```python
from build123d import *

# Parameters (mm, degrees)
SKETCH1_R                = 50
BOSS_EXTRUDE1_DEPTH      = 10
SKETCH2_R                = 20
BOSS_EXTRUDE2_DEPTH      = 280
BOSS_EXTRUDE3_START      = -10
BOSS_EXTRUDE3_DEPTH      = 10
BOSS_EXTRUDE4_DEPTH      = 10
BOSS_EXTRUDE4_DEPTH_BACK = 10
SKETCH5_R                = 20


with BuildPart() as part:
    # Sketch1 → Boss-Extrude1 (new body)
    with BuildSketch(Plane(origin=(0, 0, 0), x_dir=(1, 0, 0), z_dir=(0, 1, 0))):
        with Locations(Location((0, 0, 0), (0, 0, 270))):
            Circle(SKETCH1_R)
    extrude(amount=BOSS_EXTRUDE1_DEPTH)

    # Sketch2 → Boss-Extrude2 (add)
    with BuildSketch(Plane(origin=(0, 10, 0), x_dir=(1, 0, 0), z_dir=(0, 1, 0))):
        with Locations(Location((0, 0, 0), (0, 0, 270))):
            Circle(SKETCH2_R)
    extrude(amount=BOSS_EXTRUDE2_DEPTH)

    # Sketch4 → Boss-Extrude3 (add)
    with BuildSketch(Plane(origin=(0, 290, 0), x_dir=(1, 0, 0), z_dir=(0, 1, 0)).offset(BOSS_EXTRUDE3_START)):
        with BuildLine():
            Line((0, 20), (300, 20))
            Line((300, 20), (300, -20))
            Line((300, -20), (0, -20))
            ThreePointArc((0, -20), (-20, 0), (0, 20))
        make_face()
    extrude(amount=BOSS_EXTRUDE3_DEPTH)

    # Sketch5 → Boss-Extrude4 (add, two sides: drawn at the far end of the back side and taken through both)
    with BuildSketch(Plane(origin=(0, 290, 0), x_dir=(1, 0, 0), z_dir=(0, 1, 0)).offset(-BOSS_EXTRUDE4_DEPTH_BACK)):
        with Locations(Location((300, 0, 0), (0, 0, 270))):
            Circle(SKETCH5_R)
    extrude(amount=BOSS_EXTRUDE4_DEPTH + BOSS_EXTRUDE4_DEPTH_BACK)


solid = part.part
```
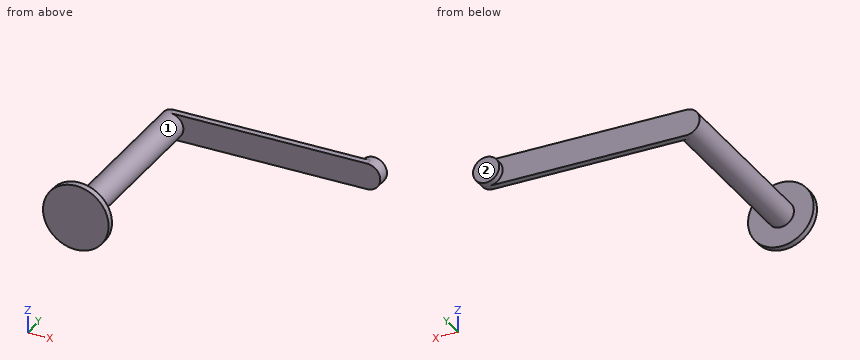
CAD build for the part. Positions are in the model's coordinates, mm. Face numbers are marked on the shaded views. A direction names the side the tool comes from. Round coordinates to 2 decimals unless told otherwise and drop trailing zeros. Loops run counter-clockwise (first coordinate to the right, second up) from the corner with the lowest first, then second, coordinate; pieces in that order, holes last. Notation, with made-up numbers: M -12.5,-36 L 16.5,-36 A20 ccw 16.5,-1 Z; hole C -38.75,81.25 d7. An arc over 180 degrees is marked long. Use a Markdown table: item, result. Add a question column.
(1) Which spindle directions (+Z, -Z, +X, -X, +Y, -Y) get a long thin tool onto all of the face, cutting with end or side? Do the marked faces 1 and 2. Say none if no direction does.
(2) Cut at B-B (y = 63.5). Give the cut face in (x, z).
(3) Cut at A-A (z = 0). Give the cut face in (x, y), and give its area (3 significant figures).
(4) Cut at C-C (x = 166). Give the cut face in (y, z).
(5) Flat gauge pins, fed straight in: pin 1 (4 mm diameter, centred on x = 177, z = 14, fed in from +Y); pin 2 (3 mm diameter, centred on x = 137, y = 284.5, fed in from +Z); pin 3 (11 mm diameter, centred on x = 142.5, y = 284.5, fed in from -Z). Where does each tip first touch, or does it go through?
(6) Drill centre lines: line 1 (Y direction, x = 25.5, z = 9); line 2 (Y direction, x = 279, z = -7); line 3 (Y direction, x = 1.5, z = -14). Where is each one in solid material? Low to high.
Geometry says:
| question | item | result |
|---|---|---|
| 1 | face 1 | none |
| 1 | face 2 | +Z, -Z, +X, -X, +Y |
| 2 | outline | C 0,0 d40 |
| 3 | outline | M -50,0 L 50,0 L 50,10 L 20,10 L 20,280 L 320,280 L 320,300 L 280,300 L 280,290 L -20,290 L -20,10 L -50,10 Z |
| 3 | area | 15,600 mm² |
| 4 | outline | M 280,-20 L 290,-20 L 290,20 L 280,20 Z |
| 5 | pin 1 | stops at y = 290 |
| 5 | pin 2 | stops at z = 20 |
| 5 | pin 3 | stops at z = -20 |
| 6 | line 1 | y = 0 to 10, 280 to 290 |
| 6 | line 2 | y = 280 to 290 |
| 6 | line 3 | y = 0 to 290 |
